Here's how the part is built. I have some questions about the finished solid (model axes, mm). A direction names the side the tool comes from. Coordinates: 2 decimals unless noted, no trailing zeros. Loops run counter-clockwise (first coordinate to the right, second up) from the corner with the lowest first, then second, coordinate; pieces in that order, holes last. Notation, with made-up numbers: (-15, 63.25) -> (17, 63.25) arc R21 cw to (17, 97.25) -> close; hole circle Ø11 at (80.5, 77.25). An arc over 180 degrees is marked (long way). Answer as a JSON object with one key per item and string values. Group by question number.
Q1. I'm going to push flat-ended pins straight in: pin 1 (2 mm diameter, centred on y = 6.5, z = 1, fed in from +X); pin 2 (1.7 mm diameter, centred on x = -0.5, y = -1, fed in from +Z); pin 3 (2.5 mm diameter, centred on x = 0, y = 0, fed in from -Z); pin 4 (2 mm diameter, centred on y = 6, z = 2, fed in from -X) (3 decimals). Where does each tip first touch, or does it pass through?
Q2. I need wall thicknesses on line 1 (Y direction, x = 0, z = 2.1); line 2 (X direction, y = -0.75, z = 3.5); line 3 (Y direction, x = -1.25, z = 1.45). Which ranges of each line are inside material? Lowest first, please.
Q3. I want a section at D-D on z = 0.3. Write out the boundary of the cut face in (x, y), then the cut area to 3 significant figures.
Q4. I want a section at C-C on z = 2.65. Write out the boundary of the cut face in (x, y).
Q5. On a 3-axis mill with a long thin cutter (end or side, diameter ignored), from which of +Z, -Z, +X, -X, +Y, -Y can I reach the whole of each face in a straight line? I mean faces 1 (the flat face through (1.25, -1.25, 0)), 2 (the cylindrical face through (-3, 0, 2)). Say none if no direction works.
Q6. Thinking about a two-plate mould opening in X: for faces 3 (the cylindrical face through (-1.73, -7.81, 2.89)), 4 (the cylindrical face through (-1.27, -0.97, 0.25)), 5 (the flat face through (3.4, 0.1, 4)), which applies, released by +X, released by -X, zero draft, split by the parting line, or undercut?
Q7. I want a section at A-A on y = 0. Write out the boundary of the cut face in (x, z), then the cut area to 3 significant figures.
```python
from build123d import *

# Parameters (mm, degrees)
F0_R     = 3
F0_R_2   = 1.6
F1_DEPTH = 0.5
F0_R_3   = 8
F2_DEPTH = 4
F3_SIZE  = 2
F4_SIZE  = 0.2


with BuildPart() as f1:
    # F0 (on Top) → F1 (new body)
    with BuildSketch(Plane.XY):
        Circle(F0_R)
        Circle(F0_R_2, mode=Mode.SUBTRACT)
    extrude(amount=F1_DEPTH)

    # F0 (on Top) → F2 (join)
    with BuildSketch(Plane.XY):
        Circle(F0_R_3)
        Circle(F0_R, mode=Mode.SUBTRACT)
    extrude(amount=F2_DEPTH)

    # F3
    f3_edges = [f1.edges().sort_by_distance(p)[0] for p in [
        (-8, 0, 0),
    ]]
    chamfer(f3_edges, length=F3_SIZE)

    # F4
    f4_edges = [f1.edges().sort_by_distance(p)[0] for p in [
        (-8, 0, 4),
        (-3, 0, 4),
        (-3, 0, 0.5),
    ]]
    chamfer(f4_edges, length=F4_SIZE)


solid = f1.part
```
Result set:
{
 "1": {"pin 1": "stops at x = 5.1", "pin 2": "stops at z = 0.5", "pin 3": "passes through", "pin 4": "stops at x = -6.245"},
 "2": {"line 1": "y = -8 to -3, 3 to 8", "line 2": "x = -7.96 to -2.9, 2.9 to 7.96", "line 3": "y = -7.34 to -2.73, 2.73 to 7.34"},
 "3": {"outline": "circle Ø12.6 at (0, 0); hole circle Ø3.2 at (0, 0)", "area": "117 mm²"},
 "4": {"outline": "circle Ø16 at (0, 0); hole circle Ø6 at (0, 0)"},
 "5": {"face 1": "-Z, +X, -X, +Y, -Y", "face 2": "+Z"},
 "6": {"face 3": "split by the parting line", "face 4": "undercut", "face 5": "zero draft"},
 "7": {"outline": "(-8, 2) -> (-6, 0) -> (-1.6, 0) -> (-1.6, 0.5) -> (-2.8, 0.5) -> (-3, 0.7) -> (-3, 3.8) -> (-3.2, 4) -> (-7.8, 4) -> (-8, 3.8) -> close; (1.6, 0) -> (6, 0) -> (8, 2) -> (8, 3.8) -> (7.8, 4) -> (3.2, 4) -> (3, 3.8) -> (3, 0.7) -> (2.8, 0.5) -> (1.6, 0.5) -> close", "area": "37.4 mm²"}
}
